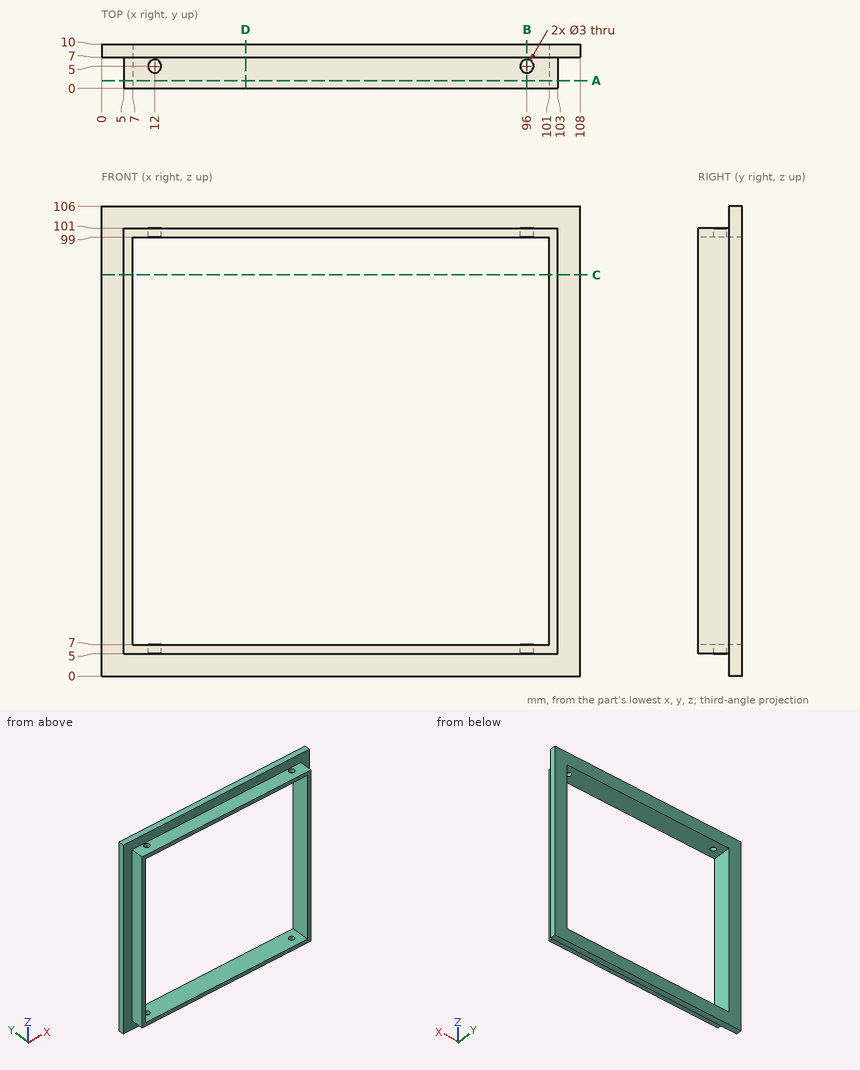
Answer from the drawing. Dimensions are ordinates in mm from the lowest x, y and z of the part. Coordinates: 2 decimals unless noted, no trailing zeros. Loops run counter-clockwise (first coordinate to the right, second up) from the corner with the lowest first, then second, coordinate; pieces in that order, holes last.
Q1. The part is cut by section D-D on x = 32.5. Write down the section's boundary in (y, z), and give its area (3 significant figures).
Q2. The part is cut by section B-B on x = 96. Write down the section's boundary in (y, z).
Q3. Consider probe 1 along X at (y, z) = (5, 6.25); probe 2 along Z at (x, y) = (99.5, 7.5); probe 3 along Z at (x, y) = (86.5, 4). Determine where each line is inside the solid, lowest interval first.
Q4. The part is cut by section C-C on z = 90.5. Write down the section's boundary in (x, y).
Q5. Each of these flat-tipped pins is pushed along its axis until it touches: pin 1 Ø2 at (x, y) = (54.5, 4.5) entering from +Z; pin 2 Ø5 at (x, y) = (96, 5) entering from +Z; pin 3 Ø5.5 at (y, z) = (3, 40) entering from +X; pin 4 Ø3.5 at (x, y) = (70.5, 3) entering from -Z. Where does it stop, or does it pass through?
Q6. The part is cut by section A-A on y = 1.75. Write down the section's boundary in (x, z), and give its area (3 significant figures).
Results below:
1. outline: (0, 5) - (7, 5) - (7, 0) - (10, 0) - (10, 7) - (0, 7) - close; (0, 99) - (10, 99) - (10, 106) - (7, 106) - (7, 101) - (0, 101) - close
1. area: 70.0 mm2
2. outline: (0, 5) - (3.5, 5) - (3.5, 7) - (0, 7) - close; (0, 99) - (3.5, 99) - (3.5, 101) - (0, 101) - close; (6.5, 5) - (7, 5) - (7, 0) - (10, 0) - (10, 7) - (6.5, 7) - close; (6.5, 99) - (10, 99) - (10, 106) - (7, 106) - (7, 101) - (6.5, 101) - close
3. probe 1: x = 5 to 10.5, 13.5 to 94.5, 97.5 to 103
3. probe 2: z = 0 to 7, 99 to 106
3. probe 3: z = 5 to 7, 99 to 101
4. outline: (0, 7) - (5, 7) - (5, 0) - (7, 0) - (7, 10) - (0, 10) - close; (101, 0) - (103, 0) - (103, 7) - (108, 7) - (108, 10) - (101, 10) - close
5. pin 1: stops at z = 101
5. pin 2: stops at z = 106
5. pin 3: stops at x = 103
5. pin 4: stops at z = 5
6. outline: (5, 5) - (103, 5) - (103, 101) - (5, 101) - close; hole (7, 7) - (101, 7) - (101, 99) - (7, 99) - close
6. area: 760 mm2
